Autodesk Fusion 360 part; units mm, degrees
sketch "Boceto1" plane through (0, 0, 0) normal (0, 0, 1) x (1, 0, 0)
  line L0 (-23.1, 5.5) -> (-23.1, -5.5)
  line L1 (-23.1, -5.5) -> (-13.1, -5.5)
  line L2 (-13.1, -5.5) -> (-2.5, -1)
  line L3 (-2.5, -1) -> (2.5, -1)
  line L4 (2.5, -1) -> (13.1, -5.5)
  line L5 (13.1, -5.5) -> (23.1, -5.5)
  line L6 (23.1, -5.5) -> (23.1, 5.5)
  line L7 (23.1, 5.5) -> (13.1, 5.5)
  line L8 (13.1, 5.5) -> (2.5, 1)
  line L9 (2.5, 1) -> (-2.5, 1)
  line L10 (-2.5, 1) -> (-13.1, 5.5)
  line L11 (-13.1, 5.5) -> (-23.1, 5.5)
  line L12 (0, -1) -> (0, 1) construction
  line L13 (-23.1, 0) -> (23.1, 0) construction
  circle A0 centre (-17.5, 0) radius 2.1
  circle A1 centre (17.5, 0) radius 2.1
  point P0 (-19.6, 0)
  point P1 (-17.5, -2.1)
  dimension "d1" = 11
  dimension "d2" = 4.2
  dimension "d3" = 5
  dimension "d4" = 3.5
  dimension "d5" = 35
  dimension "d6" = 2
  dimension "d7" = 10
  dimension "d8" = 3.4
extrude "Extruir1" add sketch "Boceto1" along normal blind 1.6
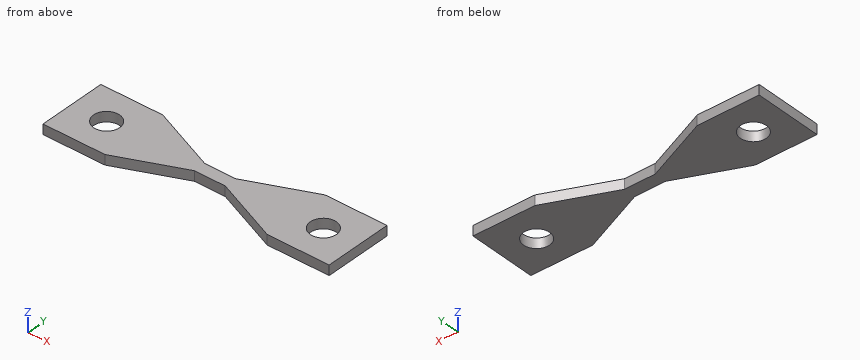
Part model, mm, in its own coordinate system. Round coordinates to 2 decimals unless told otherwise and drop trailing zeros. Write each loop counter-clockwise with the first axis right and the second up, starting at its lowest first coordinate (ties: lowest second). Pieces come first, ordered by that corner, then holes. Notation, with made-up numbers: M -9,73.5 L 5,73.5 A14 cw 5,85.5 Z; hole C 56.25,3 d10. An arc over 180 degrees is marked long. Answer as CSV lines item,"result". Start each with the question number.
1) Drop flat-ended pins along their axis: pin 1 (0.5 mm diameter, centred on x = 1, z = 0.5, fed in from +Y); pin 2 (0.8 mm diameter, centred on x = 0, z = 1, fed in from -Y). Give the stop position or say it passes through.
2) Band-saw the part on B-B (x = 17.5). List the corners of the cut face in (y, z).
3) Band-saw the part on D-D (y = -2.75). List the corners of the cut face in (x, z).
4) Band-saw the part on C-C (z = 0.55). List the corners of the cut face in (x, y).
5) Band-saw the part on A-A (y = 0). List the corners of the cut face in (x, z).
6) Drill centre lines: L1, parallel to Y at x = 17.5, z = 0.8; L2, parallel to X at y = 0.5, z = 1.1; L3, parallel to X at y = -1.75, z = 0.6. Where is each one in solid material? Low to high.
Worked out:
1,pin 1,"y = 1"
1,pin 2,"y = -1"
2,outline,"M -5.5,0 L -2.1,0 L -2.1,1.6 L -5.5,1.6 Z; M 2.1,0 L 5.5,0 L 5.5,1.6 L 2.1,1.6 Z"
3,outline,"M -23.1,0 L -6.62,0 L -6.62,1.6 L -23.1,1.6 Z; M 6.62,0 L 23.1,0 L 23.1,1.6 L 6.62,1.6 Z"
4,outline,"M -23.1,-5.5 L -13.1,-5.5 L -2.5,-1 L 2.5,-1 L 13.1,-5.5 L 23.1,-5.5 L 23.1,5.5 L 13.1,5.5 L 2.5,1 L -2.5,1 L -13.1,5.5 L -23.1,5.5 Z; hole C -17.5,0 d4.2; hole C 17.5,0 d4.2"
5,outline,"M -23.1,0 L -19.6,0 L -19.6,1.6 L -23.1,1.6 Z; M -15.4,0 L 15.4,0 L 15.4,1.6 L -15.4,1.6 Z; M 19.6,0 L 23.1,0 L 23.1,1.6 L 19.6,1.6 Z"
6,L1,"-5.5 to -2.1, 2.1 to 5.5"
6,L2,"-23.1 to -19.54, -15.46 to 15.46, 19.54 to 23.1"
6,L3,"-23.1 to -18.66, -16.34 to -4.27, 4.27 to 16.34, 18.66 to 23.1"
